from build123d import *

# Parameters (mm, degrees)
SKETCH1_W           = 25.4
SKETCH1_H           = 50.8
SKETCH1_W_2         = 19.05
SKETCH1_H_2         = 44.45
BOSS_EXTRUDE1_DEPTH = 273.05
SKETCH2_R           = 2.2479
CUT_EXTRUDE5_DEPTH  = 3.175
CUT_EXTRUDE9_START  = 3.175
SKETCH2_5_R         = 2.2479
CUT_EXTRUDE9_DEPTH  = 48.625


with BuildPart() as part:
    # Sketch1 → Boss-Extrude1 (new body, symmetric)
    with BuildSketch(Plane.XY):
        with Locations((12.7, 25.4)):
            Rectangle(SKETCH1_W, SKETCH1_H)
        with Locations((12.7, 25.4)):
            Rectangle(SKETCH1_W_2, SKETCH1_H_2, mode=Mode.SUBTRACT)
    extrude(amount=BOSS_EXTRUDE1_DEPTH, both=True)

    # Sketch2 → Cut-Extrude5 (cut)
    with BuildSketch(Plane(origin=(0, 0, 0), x_dir=(1, 0, 0), z_dir=(0, 1, 0))):
        with Locations((12.7, 260.35)):
            Circle(SKETCH2_R)
        with Locations((12.7, 234.95)):
            Circle(SKETCH2_R)
        with Locations((12.7, 209.55)):
            Circle(SKETCH2_R)
    cut_extrude5 = extrude(amount=CUT_EXTRUDE5_DEPTH, mode=Mode.SUBTRACT)

    # Sketch2<5> → Cut-Extrude9 (cut, through all)
    with BuildSketch(Plane(origin=(0, 0, 0), x_dir=(1, 0, 0), z_dir=(0, 1, 0)).offset(CUT_EXTRUDE9_START)):
        with Locations((12.7, 260.35)):
            Circle(SKETCH2_5_R)
        with Locations((12.7, 247.65)):
            Circle(SKETCH2_5_R)
        with Locations((12.7, 234.95)):
            Circle(SKETCH2_5_R)
        with Locations((12.7, 222.25)):
            Circle(SKETCH2_5_R)
        with Locations((12.7, 209.55)):
            Circle(SKETCH2_5_R)
    cut_extrude9 = extrude(amount=CUT_EXTRUDE9_DEPTH, mode=Mode.SUBTRACT)

    # Mirror3: Cut-Extrude5, Cut-Extrude9 across plane
    add(cut_extrude5.mirror(Plane.XY), mode=Mode.SUBTRACT)
    add(cut_extrude9.mirror(Plane.XY), mode=Mode.SUBTRACT)


solid = part.part
Build history of the part. All positions in model axes, mm. A direction names the side the tool comes from. Coordinates: 2 decimals unless noted, no trailing zeros. Write each loop counter-clockwise with the first axis right and the second up, starting at its lowest first coordinate (ties: lowest second). Pieces come first, ordered by that corner, then holes. Notation, with made-up numbers: (-28, -4) -> (16, -4) arc R31 cw to (16, 35) -> close; hole circle Ø4 at (45.5, 68). An arc over 180 degrees is marked (long way). Use CSV: the item, a comma, the result in double quotes. Start each with the question number.
Q1. 3-axis set-ups, long thin cutter, end or side, ignore diameter. For faces 1 (the flat face through (13, 47.625, 4)), 2 (the flat face through (2, 24, 273.05)): which of +Z, -Z, +X, -X, +Y, -Y reach the whole face in a straight line?
Q2. Cut at B-B, the plane y = 41. List the corners of the cut face in (x, z) (3 decimals).
Q3. Cut at A-A, the plane z = -64.5. List the corners of the cut face in (x, y) (3 decimals).
Q4. Pull direction Y, two halves, no side cores. Call faces 3 (the flat face through (0, 25, 4)), 4 (the flat face through (13, 0, 4)), 5 (the flat face through (13, 3.175, 4)): released by +Y, released by -Y, zero draft, split by the parting line, or undercut.
Q5. Drill centre lines: probe 1 along X at (y, z) = (4, -159) (3 decimals); probe 2 along Y at (x, z) = (15.5, -41) (3 decimals); probe 3 along X at (y, z) = (50, 222). Where is each one in solid material? Low to high.
Q6. Flat gauge pins, fed straight in: pin 1 Ø3.5 at (x, z) = (12.7, -247.65) entering from -Y; pin 2 Ø2.5 at (x, z) = (12.7, -209.55) entering from +Y; pin 3 Ø2.5 at (x, z) = (12.7, 222.25) entering from +Y (3 decimals). Where does each tip first touch, or does it go through?
Checked values:
1,face 1,"+Z, -Z"
1,face 2,"+Z, +X, -X, +Y, -Y"
2,outline,"(0, -273.05) -> (3.175, -273.05) -> (3.175, 273.05) -> (0, 273.05) -> close; (22.225, -273.05) -> (25.4, -273.05) -> (25.4, 273.05) -> (22.225, 273.05) -> close"
3,outline,"(0, 0) -> (25.4, 0) -> (25.4, 50.8) -> (0, 50.8) -> close; hole (3.175, 3.175) -> (22.225, 3.175) -> (22.225, 47.625) -> (3.175, 47.625) -> close"
4,face 3,"zero draft"
4,face 4,"released by -Y"
4,face 5,"undercut"
5,probe 1,"x = 0 to 3.175, 22.225 to 25.4"
5,probe 2,"y = 0 to 3.175, 47.625 to 50.8"
5,probe 3,"x = 0 to 10.47, 14.93 to 25.4"
6,pin 1,"stops at y = 0"
6,pin 2,"passes through"
6,pin 3,"stops at y = 3.175"
